from build123d import *

# Parameters (mm, degrees)
F1_DEPTH = 3


# Not quite as in the source:
# - a feature names something its author has since deleted; it is built from what else it names


with BuildPart() as f1:
    # F0 (on Front) → F1 (new body)
    with BuildSketch(Plane.XZ):
        Polygon((-81.04, 6), (-81.04, 0), (81.04, 0), (81.04, 6), (78.04, 6), (78.04, 2.98), (75, 2.98), (75, 6), (1.52, 6), (1.52, 2.98), (-1.52, 2.98), (-1.52, 6), (-75, 6), (-75, 2.98), (-78.04, 2.98), (-78.04, 6), align=None)
    extrude(amount=F1_DEPTH)


solid = f1.part
Here's how the part is built. I have some questions about the finished solid (model axes, mm). A direction names the side the tool comes from. Give positions to 0.01 mm unless a question says otherwise; leave off trailing zeros. Loops run counter-clockwise (first coordinate to the right, second up) from the corner with the lowest first, then second, coordinate; pieces in that order, holes last. Notation, with made-up numbers: (71, 16) -> (90, 16) arc R21 cw to (90, 51) -> close; hole circle Ø3 at (-5, -3.75). An arc over 180 degrees is marked (long way). One line per item, written item: value.
Q1. We'd pull the mould along X, two halves only. Please class faces 3 (the face through (-81.04, -1, 3)), 4 (the face through (75, -1, 4)), 5 (the face through (-1, -1, 0)): pulls with the +X half, pulls with the -X half, needs draft (parallel to the pull), parting line crosses it, or undercut.
Answers follow:
face 3: pulls with the -X half
face 4: undercut
face 5: needs draft
Q2. Suppose I cut it at A-A on z = 4.6. Please give me the cut outline in (x, y), then the cut area to 3 significant figures.
Answers follow:
outline: (-81.04, -3) -> (-78.04, -3) -> (-78.04, 0) -> (-81.04, 0) -> close; (-75, -3) -> (-1.52, -3) -> (-1.52, 0) -> (-75, 0) -> close; (1.52, -3) -> (75, -3) -> (75, 0) -> (1.52, 0) -> close; (78.04, -3) -> (81.04, -3) -> (81.04, 0) -> (78.04, 0) -> close
area: 459 mm^2
Q3. I'm going to push a flat-ended pin straight in: pin 1 Ø1.5 at (x, y) = (0.5, -1.5) entering from +Z. Where does the tip first touch, or does it pass through?
Answers follow:
pin 1: z = 2.98
Q4. Suppose I cut it at B-B on y = -2.35. Please give me the cut outline in (x, z), then the cut area to 3 significant figures.
Answers follow:
outline: (-81.04, 0) -> (81.04, 0) -> (81.04, 6) -> (78.04, 6) -> (78.04, 2.98) -> (75, 2.98) -> (75, 6) -> (1.52, 6) -> (1.52, 2.98) -> (-1.52, 2.98) -> (-1.52, 6) -> (-75, 6) -> (-75, 2.98) -> (-78.04, 2.98) -> (-78.04, 6) -> (-81.04, 6) -> close
area: 945 mm^2
Q5. On a 3-axis mill with a long thin cutter (end or side, diameter ignored), from which of +Z, -Z, +X, -X, +Y, -Y can I reach the whole of each face in a straight line? I mean faces 1 (the face through (-38, -1, 6)), 2 (the face through (-78.04, -1, 4)). Say none if no direction works.
Answers follow:
face 1: +Z, +X, -X, +Y, -Y
face 2: +Z, +Y, -Y
Q6. If I drill on line 1 along X through (y, z) = (-1.2, 3.3), over which ranges is the centre line in solid material (lowest first)?
Answers follow:
line 1: -81.04 to -78.04, -75 to -1.52, 1.52 to 75, 78.04 to 81.04
